from build123d import *

# Parameters (mm, degrees)
F0_W     = 100
F0_H     = 150
F1_DEPTH = 10


with BuildPart() as f1:
    # F0 (on Front) → F1 (new body)
    with BuildSketch(Plane.XZ):
        Rectangle(F0_W, F0_H)
        Polygon((-30, -55), (-30, 44.558363), (24.304562, -55), align=None, mode=Mode.SUBTRACT)
        Polygon((-24.304562, 55), (30, 55), (30, -44.558363), align=None, mode=Mode.SUBTRACT)
    extrude(amount=F1_DEPTH)


solid = f1.part
CAD build for the part. Positions are in the model's coordinates, mm. A direction names the side the tool comes from. Coordinates: 2 decimals unless noted, no trailing zeros. Loops run counter-clockwise (first coordinate to the right, second up) from the corner with the lowest first, then second, coordinate; pieces in that order, holes last. Notation, with made-up numbers: (-24.5, 77) - (23.5, 77) arc R21 ccw to (23.5, 90) - close; hole circle Ø5 at (-15.75, -10.75). An arc over 180 degrees is marked (long way). Write item = value, one per line. Start each with the question number.
Q1. Cut at C-C, the plane z = -2. List the corners of the cut face in (x, y).
Q2. Pull direction X, two halves, no side cores. Call faces 1 (the flat face through (-1, -5, 75)), 2 (the flat face through (50, -5, -1)), 3 (the flat face through (-30, -5, -6)): pulls with the +X half, pulls with the -X half, needs draft (parallel to the pull), parting line crosses it, or undercut.
Q3. Drill centre lines: L1, parallel to Z at x = -3, y = -6.25; L2, parallel to X at y = -4.25, z = 40.5; L3, parallel to X at y = -1.5, z = -28. Where is each one in solid material? Low to high.
Q4. Which spindle directions (+Z, -Z, +X, -X, +Y, -Y) get a long thin tool onto all of the face, cutting with end or side? Do faces 4 (the flat face through (-50, -5, -1)), 5 (the flat face through (-3.23, -4.93, -4.52)). Say none if no direction does.
Q5. Cut at B-B, the plane x = 28. List the corners of the cut face in (y, z), then the cut area to 3 significant figures.
Q6. Flat gauge pin, fed straight in: pin 1 Ø2 at (x, z) = (-2, -53.5) entering from +Y. Where does the tip first touch, or does it go through?
Q7. Cut at A-A, the plane y = -2.75. List the corners of the cut face in (x, z), then the cut area to 3 significant figures.
Computed:
q1.outline = (-50, -10) - (-30, -10) - (-30, 0) - (-50, 0) - close; (-4.6, -10) - (6.79, -10) - (6.79, 0) - (-4.6, 0) - close; (30, -10) - (50, -10) - (50, 0) - (30, 0) - close
q2.face_1 = needs draft
q2.face_2 = pulls with the +X half
q2.face_3 = undercut
q3.L1 = -75 to -55, -4.94 to 15.94, 55 to 75
q3.L2 = -50 to -30, -27.79 to -16.4, 30 to 50
q3.L3 = -50 to -30, 9.58 to 20.97, 30 to 50
q4.face_4 = +Z, -Z, -X, +Y, -Y
q4.face_5 = +Y, -Y
q5.outline = (-10, -75) - (0, -75) - (0, -40.89) - (-10, -40.89) - close; (-10, 55) - (0, 55) - (0, 75) - (-10, 75) - close
q5.area = 541 mm²
q6.pin_1 = through
q7.outline = (-50, -75) - (50, -75) - (50, 75) - (-50, 75) - close; hole (-30, -55) - (24.3, -55) - (-30, 44.56) - close; hole (-24.3, 55) - (30, -44.56) - (30, 55) - close
q7.area = 9,590 mm²
